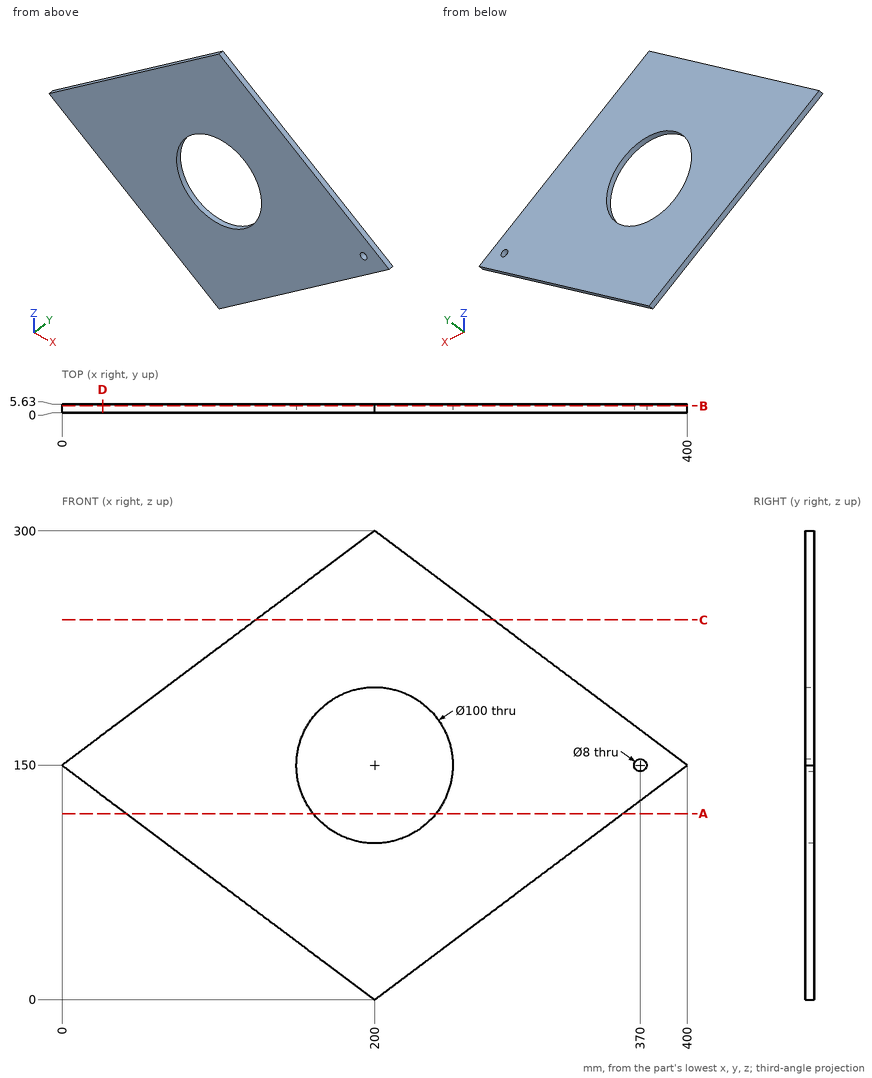
Check sheet for the drawn part. Datum: minimum x, y, z corner. Units: mm. Give positions to 0.01 mm unless a question says otherwise; leave off trailing zeros. Write each loop counter-clockwise with the first axis right and the second up, starting at its lowest first coordinate (ties: lowest second). Pieces come first, ordered by that corner, then holes.
(1) Gauge pin test, flat ends, axial feed: pin 1 (1.5 mm diameter, centred on y = 1.5, z = 78.5, fed in from +X); pin 2 (1 mm diameter, centred on x = 169, y = 3.5, fed in from -Z) (3 decimals); pin 3 (2 mm diameter, centred on y = 0.5, z = 167.5, fed in from -X); pin 4 (2 mm diameter, centred on x = 207.5, z = 73.5, fed in from -Y). Record the tip position at first contact, or that the pin passes through.
(2) Cross-section at A-A (z = 119). Enter the section's corners in (x, y), plus the area to 3 significant figures.
(3) Material ranges on line 1 (X direction, y = 3.25, z = 150); line 2 (Z direction, x = 370, y = 1.45); line 3 (X direction, y = 3.5, z = 149.5), recorded low to high.
(4) Cross-section at C-C (z = 243). Enter the section's corners in (x, y).
(5) Cross-section at B-B (y = 4.4). Enter the section's corners in (x, z), plus the area to 3 significant figures.
(6) Cross-section at D-D (x = 26). Enter the section's corners in (y, z).
Worked out:
1. pin 1: stops at x = 305.67
1. pin 2: stops at z = 22.875
1. pin 3: stops at x = 22
1. pin 4: stops at y = 0
2. outline: (41.33, 0) - (160.77, 0) - (160.77, 5.63) - (41.33, 5.63) - close; (239.23, 0) - (358.67, 0) - (358.67, 5.63) - (239.23, 5.63) - close
2. area: 1,340 mm2
3. line 1: x = 0 to 150, 250 to 366, 374 to 400
3. line 2: z = 127.5 to 146, 154 to 172.5
3. line 3: x = 0.67 to 150, 250 to 366.03, 373.97 to 399.33
4. outline: (124, 0) - (276, 0) - (276, 5.63) - (124, 5.63) - close
5. outline: (0, 150) - (200, 0) - (400, 150) - (200, 300) - close; hole circle Ø100 at (200, 150); hole circle Ø8 at (370, 150)
5. area: 52,100 mm2
6. outline: (0, 130.5) - (5.63, 130.5) - (5.63, 169.5) - (0, 169.5) - close
